```python
from build123d import *

# Parameters (mm, degrees)
SKETCH_A01_2_R     = 6.849979581
SKETCH_A01_2_R_2   = 6.85
SKETCH_A01_2_W     = 10
SKETCH_A01_2_H     = 10
EXTRUDE1_DEPTH     = 250
CUT_EXTRUDE1_DEPTH = 251
CIRPATTERN1_COUNT  = 2
CUT_EXTRUDE2_DEPTH = 251
CUT_EXTRUDE3_DEPTH = 251
CIRPATTERN2_COUNT  = 2
CIRPATTERN2_ANGLE  = 270
CIRPATTERN3_COUNT  = 2
CIRPATTERN3_ANGLE  = 90


with BuildPart() as part:
    # Sketch A01-2 → Extrude1 (new body)
    with BuildSketch(Plane.XY):
        Polygon((-16.5, -36), (-16.5, -34.5), (-15.863961, -34.5), (-10.14602885, -28.78206785), (-10.14602885, -21.21793215), (-15.863961, -15.5), (-16.5, -15.5), (-16.5, -14), (-21, -14), (-21, -21), (-25, -21), (-25, -4), (-21, -4), (-21, -11), (-16.5, -11), (-16.5, -9.5), (-15.863961, -9.5), (-10.14602885, -3.78206785), (-10.14602885, 3.78206785), (-15.863961, 9.5), (-16.5, 9.5), (-16.5, 11), (-21, 11), (-21, 4), (-25, 4), (-25, 21), (-21, 21), (-21, 14), (-16.5, 14), (-16.5, 15.5), (-15.863961, 15.5), (-10.14602885, 21.21793215), (-10.14602885, 28.78206785), (-15.863961, 34.5), (-16.5, 34.5), (-16.5, 36), (-21, 36), (-21, 29), (-25, 29), (-25, 50), (-4, 50), (-4, 46), (-11, 46), (-11, 41.5), (-9.5, 41.5), (-9.5, 40.863961), (-3.78206785, 35.14602885), (3.78206785, 35.14602885), (9.5, 40.863961), (9.5, 41.5), (11, 41.5), (11, 46), (4, 46), (4, 50), (25, 50), (25, 29), (21, 29), (21, 36), (16.5, 36), (16.5, 34.5), (15.863961, 34.5), (10.14602885, 28.78206785), (10.14602885, 21.21793215), (15.863961, 15.5), (16.5, 15.5), (16.5, 14), (21, 14), (21, 21), (25, 21), (25, 4), (21, 4), (21, 11), (16.5, 11), (16.5, 9.5), (15.863961, 9.5), (10.14602885, 3.78206785), (10.14602885, -3.78206785), (15.863961, -9.5), (16.5, -9.5), (16.5, -11), (21, -11), (21, -4), (25, -4), (25, -21), (21, -21), (21, -14), (16.5, -14), (16.5, -15.5), (15.863961, -15.5), (10.14602885, -21.21793215), (10.14602885, -28.78206785), (15.863961, -34.5), (16.5, -34.5), (16.5, -36), (21, -36), (21, -29), (25, -29), (25, -50), (4, -50), (4, -46), (11, -46), (11, -41.5), (9.5, -41.5), (9.5, -40.863961), (3.78206785, -35.14602885), (-3.78206785, -35.14602885), (-9.5, -40.863961), (-9.5, -41.5), (-11, -41.5), (-11, -46), (-4, -46), (-4, -50), (-25, -50), (-25, -29), (-21, -29), (-21, -36), align=None)
        Circle(SKETCH_A01_2_R, mode=Mode.SUBTRACT)
        with Locations((0, -25)):
            Circle(SKETCH_A01_2_R_2, mode=Mode.SUBTRACT)
        with Locations((0, 25)):
            Circle(SKETCH_A01_2_R, mode=Mode.SUBTRACT)
        with Locations((-18, -43)):
            Rectangle(SKETCH_A01_2_W, SKETCH_A01_2_H, mode=Mode.SUBTRACT)
        with Locations((18, -43)):
            Rectangle(SKETCH_A01_2_W, SKETCH_A01_2_H, mode=Mode.SUBTRACT)
        with Locations((-18, 43)):
            Rectangle(SKETCH_A01_2_W, SKETCH_A01_2_H, mode=Mode.SUBTRACT)
        with Locations((18, 43)):
            Rectangle(SKETCH_A01_2_W, SKETCH_A01_2_H, mode=Mode.SUBTRACT)
    extrude(amount=-EXTRUDE1_DEPTH)

    # Sketch1 → Cut-Extrude1 (cut, through all)
    with BuildSketch(Plane.XY):
        with BuildLine():
            Line((-7.258795353, 17.320361918), (-12.614234198, 11.855428431))
            Line((-12.614234198, 11.855428431), (-12.614234198, 11.051418253))
            Line((-12.614234198, 11.051418253), (-7.258795353, 5.803280231))
            ThreePointArc((-7.258795353, 5.803280231), (-5.094968204, 7.490334338), (-2.563122733, 8.547716957))
            Line((-2.563122733, 8.547716957), (-1.967487438, 6.56134235))
            ThreePointArc((-1.967487438, 6.56134235), (0.214842487, 6.846609596), (2.374993487, 6.425077913))
            Line((2.374993487, 6.425077913), (2.972164568, 8.497096186))
            ThreePointArc((2.972164568, 8.497096186), (5.403413421, 7.442330952), (7.485963159, 5.803280231))
            Line((7.485963159, 5.803280231), (12.841402004, 11.051418253))
            Line((12.841402004, 11.051418253), (12.841402004, 11.855428431))
            Line((12.841402004, 11.855428431), (7.485963159, 17.320361918))
            ThreePointArc((7.485963159, 17.320361918), (0.113583903, 14.310231562), (-7.258795353, 17.320361918))
        make_face()
    cut_extrude1 = extrude(amount=-CUT_EXTRUDE1_DEPTH, mode=Mode.SUBTRACT)

    # CirPattern1: Cut-Extrude1 ×2 about axis
    cirpattern1_axis = Axis((0, 0, 0), (0, 0, 1))
    for i in range(1, CIRPATTERN1_COUNT):
        add(cut_extrude1.rotate(cirpattern1_axis, i * 360 / CIRPATTERN1_COUNT), mode=Mode.SUBTRACT)

    # Sketch2 → Cut-Extrude2 (cut, through all)
    with BuildSketch(Plane.XY):
        Polygon((-16.419523035, 38), (-9.694317474, 31.274794439), (-6.274794439, 34.694317474), (-13, 41.419523035), align=None)
    cut_extrude2 = extrude(amount=-CUT_EXTRUDE2_DEPTH, mode=Mode.SUBTRACT)

    # Sketch3 → Cut-Extrude3 (cut, through all)
    with BuildSketch(Plane.XY):
        Polygon((-16.519090004, -38), (-9.847797296, -31.328707292), (-6.301034305, -34.875470283), (-13, -41.574435978), align=None)
    cut_extrude3 = extrude(amount=-CUT_EXTRUDE3_DEPTH, mode=Mode.SUBTRACT)

    # CirPattern2: Cut-Extrude2 ×2 about axis
    cirpattern2_axis = Axis((0, 25, 0), (0, 0, 1))
    for i in range(1, CIRPATTERN2_COUNT):
        add(cut_extrude2.rotate(cirpattern2_axis, i * CIRPATTERN2_ANGLE / (CIRPATTERN2_COUNT - 1)), mode=Mode.SUBTRACT)

    # CirPattern3: Cut-Extrude3 ×2 about axis
    cirpattern3_axis = Axis((0, -25, 0), (0, 0, 1))
    for i in range(1, CIRPATTERN3_COUNT):
        add(cut_extrude3.rotate(cirpattern3_axis, i * CIRPATTERN3_ANGLE / (CIRPATTERN3_COUNT - 1)), mode=Mode.SUBTRACT)


solid = part.part
```
CAD build for the part. Positions are in the model's coordinates, mm. A direction names the side the tool comes from. Give positions to 0.01 mm unless a question says otherwise; leave off trailing zeros. Write each loop counter-clockwise with the first axis right and the second up, starting at its lowest first coordinate (ties: lowest second). Pieces come first, ordered by that corner, then holes. Notation, with made-up numbers: M 40,12 L 91,12 A26 cw 91,35 Z; hole C -12,-12.75 d7. An arc over 180 degrees is marked long. Return JSON: item names as keys, results as strings. Group by question number.
(1) Band-saw the part on A-A (y = -25). Give the cut face in (x, z).
(2) Band-saw the part on B-B (z = -105). State how many separate pieces and enclosed holes the cut face has, and give its area (3 significant figures).
(3) Flat gauge pin, fed straight in: pin 1 Ø1 at (y, z) = (-1.5, -126.5) entering from +X. Where does the tip first touch, or does it go through?
(4) Drill centre lines: L1, parallel to Y at x = 0, z = -176; L2, parallel to Y at x = 21.5, z = -206.5; L3, parallel to X at y = 43.5, z = -219. Where is each one in solid material? Low to high. Write a range as [from, to].
(5) 3-axis set-ups, long thin cutter, end or side, ignore diameter. For faces 1 (the face through (-13.23, -34.71, -123.25)), 2 (the face through (15, -50, -123)): which of +Z, -Z, +X, -X, +Y, -Y reach the whole face in a straight line?
(6) Mould opens along X. For faces 3 (the face through (-7, 0, -250)), 4 (the face through (-13, -45, -123)), 5 (the face through (-19, 14, -123)) say: pulls with the +X half, pulls with the -X half, needs draft (parallel to the pull), parting line crosses it, or undercut.
Entries:
{
 "1": {"outline": "M -10.15,-250 L -6.85,-250 L -6.85,0 L -10.15,0 Z; M 6.85,-250 L 10.15,-250 L 10.15,0 L 6.85,0 Z"},
 "2": {"separate pieces": "1", "enclosed holes": "7", "area": "1,870 mm^2"},
 "3": {"pin 1": "stops at x = 10.15"},
 "4": {"L1": "y = [-35.15, -31.85], [-18.15, -14.31], [14.31, 18.15], [31.85, 35.15]", "L2": "y = [-50, -48], [-38, -29], [-21, -4], [4, 21], [29, 38], [48, 50]", "L3": "x = [-25, -23], [-13, -11], [11, 13], [23, 25]"},
 "5": {"face 1": "+Z, -Z", "face 2": "+Z, -Z, +X, -X, -Y"},
 "6": {"face 3": "needs draft", "face 4": "undercut", "face 5": "undercut"}
}
